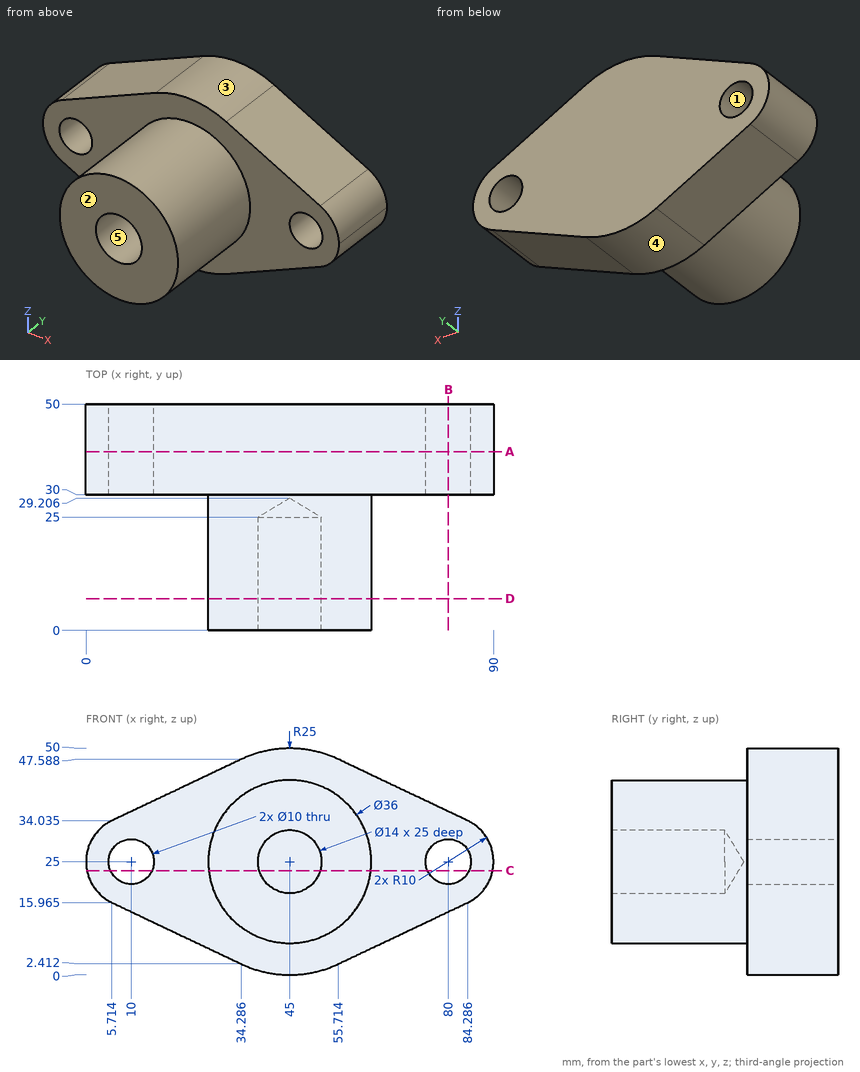
Geometry check sheet. Reference: drawing and pictorial views, mm from the part's lowest x, y, z. A direction names the side the tool comes from. Give positions to 0.01 mm unless a question says otherwise; leave off trailing zeros. Write each loop counter-clockwise with the first axis right and the second up, starting at its lowest first coordinate (ties: lowest second). Pieces come first, ordered by that corner, then holes. Notation, with made-up numbers: M 67.5,-25 L 108.5,-25 A19 ccw 108.5,-12 Z; hole C 26.5,51 d10. An arc over 180 degrees is marked long. Answer as CSV lines item,"result". Start each with the question number.
Q1. Section check B-B, the plane x = 80. Record the cut outline in (y, z).
Q2. Section check D-D, the plane y = 7. Record the cut outline in (x, z).
Q3. Tool access check on the marked faces 4 and 5. Record the directions out of +Z, -Z, +X, -X, +Y, -Y that give a thin tool (end or side, any length) a straight path to the whole face; none if there is none.
Q4. Section check C-C, the plane z = 23. Give the number of separate pieces and of enclosed holes in the cut face, then the cut area to 3 significant figures.
Q5. Material ranges on L1, parallel to Z at x = 45, y = 13; L2, parallel to Y at x = 68, z = 32; L3, parallel to Z at x = 80, y = 39.25, recorded low to high.
Q6. Go/stop test with flat-tipped pins: pin 1 (9 mm diameter, centred on x = 10, z = 25, fed in from -Y); pin 2 (1 mm diameter, centred on y = 23, z = 36, fed in from +X); pin 3 (8 mm diameter, centred on x = 35.5, y = 29, fed in from +Z); pin 4 (6 mm diameter, centred on y = 19.5, z = 11.5, fed in from -X). Record where each tip stops, or that it passes through.
Q7. Section check A-A, the plane y = 39.5. Record the cut outline in (x, z) (1 decimal), then the cut area to 3 significant figures.
Q8. Release check for a two-part mould opening along Z. For the marked faces 1, 2 and 3 record: pulls with the +Z half, pulls with the -Z half, needs draft (parallel to the pull), parting line crosses it, or undercut.
Geometry says:
1,outline,"M 30,13.93 L 50,13.93 L 50,20 L 30,20 Z; M 30,30 L 50,30 L 50,36.07 L 30,36.07 Z"
2,outline,"C 45,25 d36; hole C 45,25 d14"
3,face 4,"-Z, +Y, -Y"
3,face 5,"-Y"
4,separate pieces,"3"
4,enclosed holes,"0"
4,area,"2,140 mm^2"
5,L1,"7 to 18, 32 to 43"
5,L2,"30 to 50"
5,L3,"13.93 to 20, 30 to 36.07"
6,pin 1,"through"
6,pin 2,"x = 59.62"
6,pin 3,"z = 49.36"
6,pin 4,"x = 30.38"
7,outline,"M 5.7,16 L 34.3,2.4 A25 ccw 55.7,2.4 L 84.3,16 A10 ccw 84.3,34 L 55.7,47.6 A25 ccw 34.3,47.6 L 5.7,34 A10 ccw Z; hole C 10,25 d10; hole C 80,25 d10"
7,area,"2,840 mm^2"
8,face 1,"undercut"
8,face 2,"needs draft"
8,face 3,"pulls with the +Z half"
